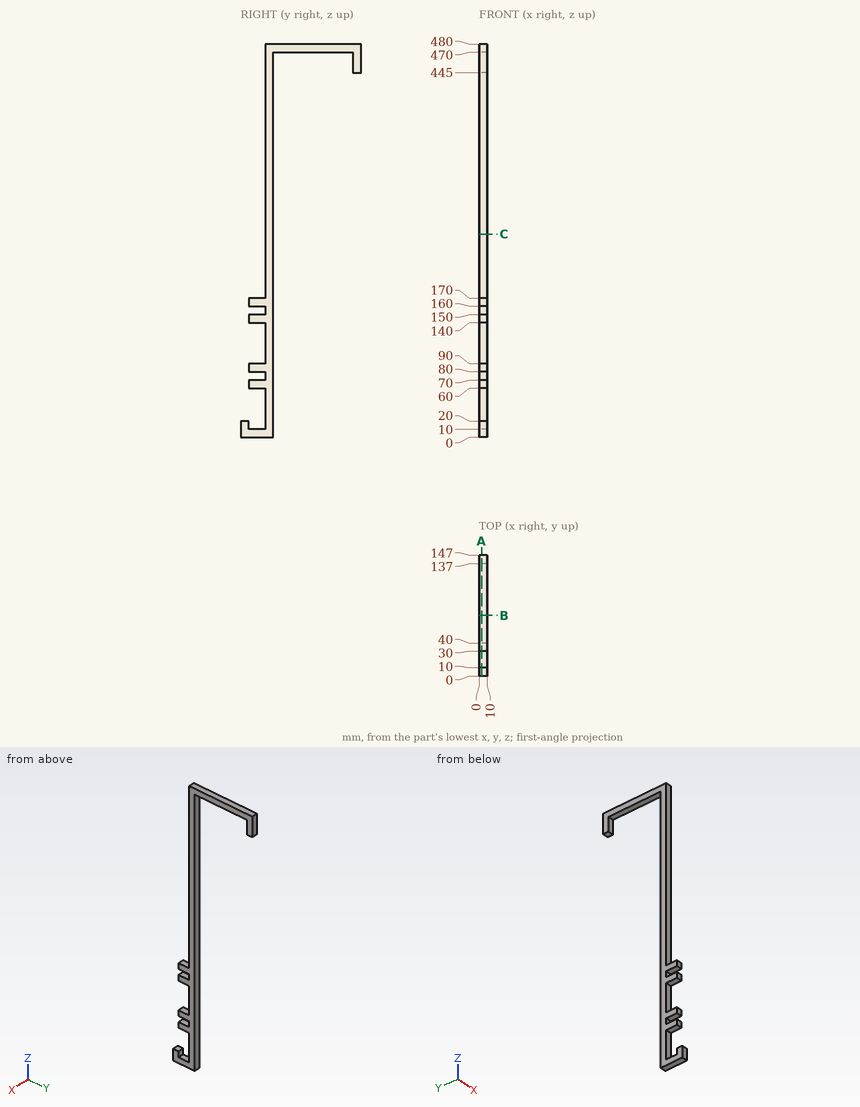
Drawing for the job (mm, zero at the part's lowest x, y, z). Round coordinates to 2 decimals unless told otherwise and drop trailing zeros. Loops run counter-clockwise (first coordinate to the right, second up) from the corner with the lowest first, then second, coordinate; pieces in that order, holes last. Notation, with made-up numbers: (-2.75, -34) - (14.25, -34) arc R29 ccw to (14.25, 0) - close; hole circle Ø4 at (-38.75, 39). An arc over 180 degrees is marked (long way). Return JSON: item names as keys, results as strings. Group by question number.
Q1. Band-saw the part on C-C on z = 248. Give the cut face in (x, y), plus the area to 3 significant figures.
Q2. Band-saw the part on B-B on y = 74. Give the cut face in (x, z).
Q3. Drill centre lines: line 1 along Z through (x, y) = (8.75, 22); line 2 along Y through (x, z) = (9, 84); line 3 along Y through (x, z) = (6, 411.5). Where is each one in solid material? Low to high. Write a range as [from, to].
Q4. Band-saw the part on A-A on x = 3. Give the cut face in (y, z), plus the area to 3 significant figures.
Q5. Flat gauge pins, fed straight in: pin 1 Ø5 at (x, y) = (5.5, 22) entering from +Z; pin 2 Ø5 at (x, z) = (3, 110.5) entering from -Y; pin 3 Ø5 at (x, z) = (3, 143.5) entering from -Y. Where does each tip first touch, or does it go through?
Solutions:
{
 "1": {"outline": "(0, 30) - (10, 30) - (10, 40) - (0, 40) - close", "area": "100 mm^2"},
 "2": {"outline": "(0, 470) - (10, 470) - (10, 480) - (0, 480) - close"},
 "3": {"line 1": "z = [0, 10], [60, 70], [80, 90], [140, 150], [160, 170]", "line 2": "y = [10, 40]", "line 3": "y = [30, 40]"},
 "4": {"outline": "(0, 0) - (40, 0) - (40, 470) - (137, 470) - (137, 445) - (147, 445) - (147, 480) - (30, 480) - (30, 170) - (10, 170) - (10, 160) - (30, 160) - (30, 150) - (10, 150) - (10, 140) - (30, 140) - (30, 90) - (10, 90) - (10, 80) - (30, 80) - (30, 70) - (10, 70) - (10, 60) - (30, 60) - (30, 10) - (10, 10) - (10, 20) - (0, 20) - close", "area": "7,320 mm^2"},
 "5": {"pin 1": "stops at z = 170", "pin 2": "stops at y = 30", "pin 3": "stops at y = 10"}
}
